Answer from the drawing. Dimensions are ordinates in mm from the lowest x, y and z of the part. A direction names the side the tool comes from. Give positions to 0.01 mm unless a question says otherwise; leave off trailing zeros. Put each result on its own line as item: value. Start each with the question number.
1. For a pull along Z with two mould halves and no side action, classify the marked faces 4, 5, 6 and 7 as released by +Z, released by -Z, zero draft, split by the parting line, or undercut.
2. For the marked faces 1, 2 and 3, determine the directions among +Z, -Z, +X, -X, +Y, -Y from which every point of the face is accessible in a straight line to the end or side of a thin tool.
3. Given pin 1 Ø2 at (x, y) = (5, 2) entering from +Z, flat-ended and moving along its own axis, determine where the tip first touches the part or whether it passes through.
4. Consider L1, parallel to Y at x = 3.5, z = 0.5 (3 decimals); L2, parallel to Z at x = 2.5, y = 4; L3, parallel to Z at x = 2, y = 6. Determine where each line is inside the solid, lowest interval first. Write a range as from..to.
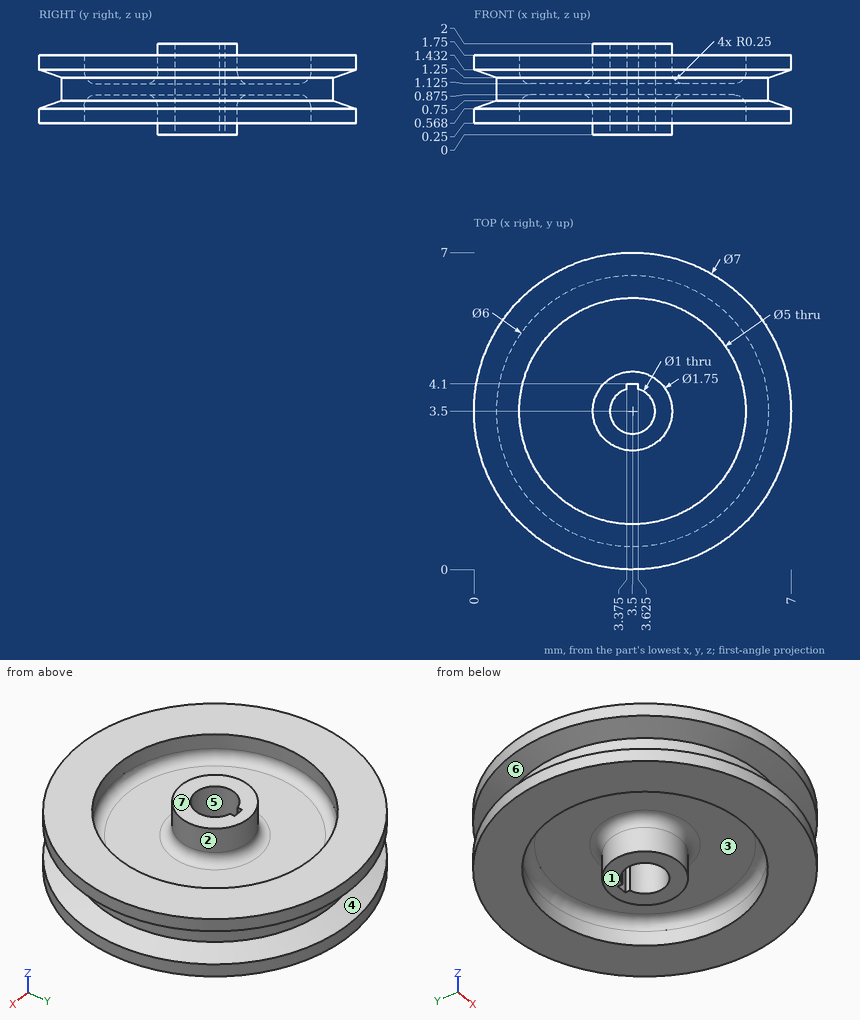
Return value:
1. face 4: undercut
1. face 5: zero draft
1. face 6: undercut
1. face 7: released by +Z
2. face 1: -Z, +X, -X, +Y, -Y
2. face 2: +Z
2. face 3: -Z
3. pin 1: stops at z = 1.75
4. L1: y = 0..1, 2.625..3, 4.1..4.375, 6..7
4. L2: z = 0.87..1.13
4. L3: z = 0.25..1.75
